Input: dimensioned drawing with shaded views. Units: mm. Origin: part minimum x, y, z. Give positions to 0.01 mm unless a question says otherwise; leave off trailing zeros. Order: outer loops, then holes, each group sorted by start corner. A loop starts at its lowest first (then second) coordinate and runs counter-clockwise, first axis right, second up.
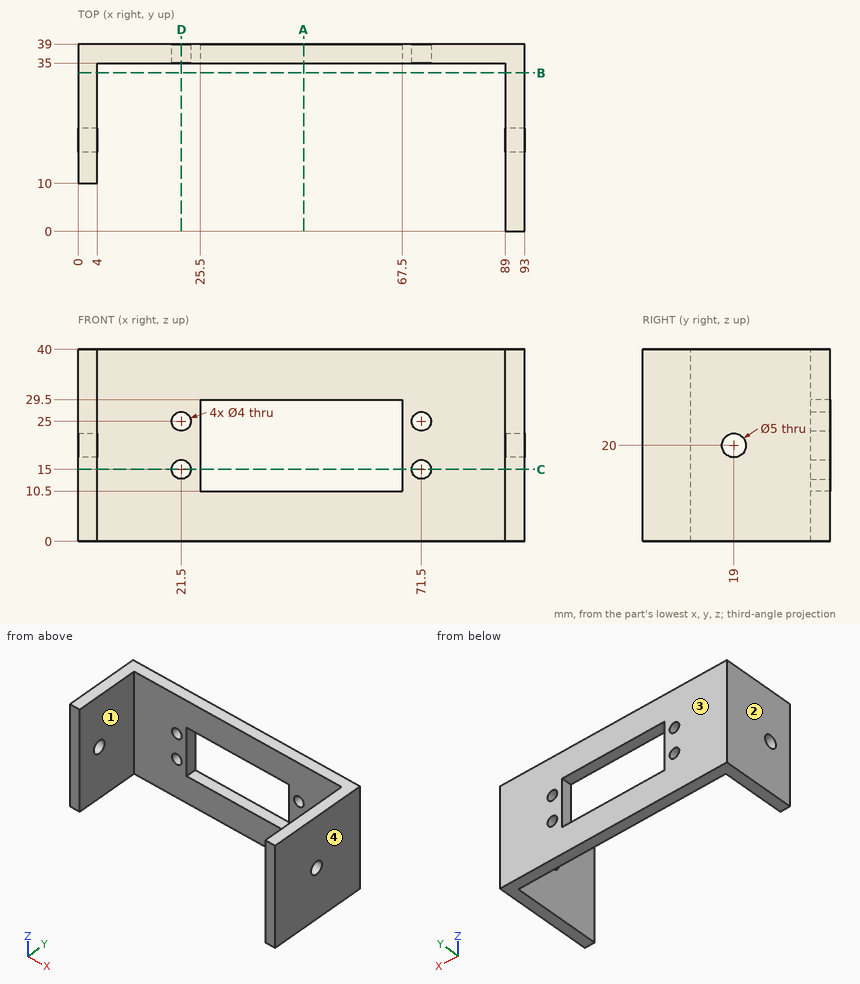
1) Section query A-A, the plane x = 47. Return the cut outline in (y, z), and give its area (3 significant figures).
Report:
outline: (35, 0) - (39, 0) - (39, 10.5) - (35, 10.5) - close; (35, 29.5) - (39, 29.5) - (39, 40) - (35, 40) - close
area: 84.0 mm2
2) Section query D-D, the plane x = 21.5. Return the cut outline in (y, z), and give its area (3 significant figures).
Report:
outline: (35, 0) - (39, 0) - (39, 13) - (35, 13) - close; (35, 17) - (39, 17) - (39, 23) - (35, 23) - close; (35, 27) - (39, 27) - (39, 40) - (35, 40) - close
area: 128 mm2
3) Section query C-C, the plane z = 15. Return the cut outline in (x, y), and give its area (3 significant figures).
Report:
outline: (0, 10) - (4, 10) - (4, 35) - (19.5, 35) - (19.5, 39) - (0, 39) - close; (23.5, 35) - (25.5, 35) - (25.5, 39) - (23.5, 39) - close; (67.5, 35) - (69.5, 35) - (69.5, 39) - (67.5, 39) - close; (73.5, 35) - (89, 35) - (89, 0) - (93, 0) - (93, 39) - (73.5, 39) - close
area: 412 mm2
4) Section query B-B, the plane y = 33. Return the cut outline in (x, z).
Report:
outline: (0, 0) - (4, 0) - (4, 40) - (0, 40) - close; (89, 0) - (93, 0) - (93, 40) - (89, 40) - close
5) Material intervals for L1, parallel to X at y = 37.1, z = 25; L2, parallel to Y at x = 2.25, z = 20; L3, parallel to X at y = 26, z = 34.5, sorted ascending.
Report:
L1: x = 0 to 19.5, 23.5 to 25.5, 67.5 to 69.5, 73.5 to 93
L2: y = 10 to 16.5, 21.5 to 39
L3: x = 0 to 4, 89 to 93
6) Pin query (flat end, axial travel): pin 1 (3 mm diameter, centred on y = 19, z = 20, fed in from -X); pin 2 (2 mm diameter, centred on x = 19, z = 17, fed in from -Y); pin 3 (3 mm diameter, centred on x = 1.5, z = 16, fed in from -Y). Return the tip coordinate at first contact, or that it passes through.
Report:
pin 1: passes through
pin 2: stops at y = 35
pin 3: stops at y = 10
7) Draft query along X for the marked faces 1, 2, 3 and 4. Return one class per face: +X half, -X half, draft (parallel to the pull), parting line (faces both ways), or undercut.
Report:
face 1: undercut
face 2: -X half
face 3: draft
face 4: +X half
